Could you check a few things on this model? Use its own coordinates, in mm. Round coordinates to 2 decimals unless told otherwise and drop trailing zeros. Loops run counter-clockwise (first coordinate to the right, second up) from the corner with the lowest first, then second, coordinate; pieces in that order, holes last. Notation, with made-up numbers: (37, 42) - (65, 42) arc R16 cw to (65, 57) - close; hole circle Ø3 at (-23.75, -22). An arc over 180 degrees is marked (long way). Use one line per item in the form item = value.
```python
from build123d import *

# Parameters (mm, degrees)
SKETCH1_R           = 40.64
SKETCH1_R_2         = 27.686
SKETCH1_R_3         = 3.556
SKETCH1_R_4         = 2.794
BOSS_EXTRUDE1_DEPTH = 2.794
SKETCH2_W           = 3.048
SKETCH2_H           = 48.134172809
CUT_EXTRUDE1_DEPTH  = 14.097


with BuildPart() as part:
    # Sketch1 → Boss-Extrude1 (new body)
    with BuildSketch(Plane.XY):
        Circle(SKETCH1_R)
        Circle(SKETCH1_R_2, mode=Mode.SUBTRACT)
        with Locations((0, 34.036)):
            Circle(SKETCH1_R_3, mode=Mode.SUBTRACT)
        with Locations((34.036, 0)):
            Circle(SKETCH1_R_3, mode=Mode.SUBTRACT)
        with Locations((0, -34.036)):
            Circle(SKETCH1_R_3, mode=Mode.SUBTRACT)
        with Locations((-34.036, 0)):
            Circle(SKETCH1_R_3, mode=Mode.SUBTRACT)
        with Locations((24.067086404, 24.067086404)):
            Circle(SKETCH1_R_4, mode=Mode.SUBTRACT)
        with Locations((24.067086404, -24.067086404)):
            Circle(SKETCH1_R_4, mode=Mode.SUBTRACT)
        with Locations((-24.067086404, -24.067086404)):
            Circle(SKETCH1_R_4, mode=Mode.SUBTRACT)
        with Locations((-24.067086404, 24.067086404)):
            Circle(SKETCH1_R_4, mode=Mode.SUBTRACT)
    extrude(amount=BOSS_EXTRUDE1_DEPTH)

    # Sketch2 → Cut-Extrude1 (cut)
    with BuildSketch(Plane.XY.offset(2.794)):
        with Locations((-24.067086404, 24.067086405)):
            Rectangle(SKETCH2_W, SKETCH2_H)
    extrude(amount=-CUT_EXTRUDE1_DEPTH, mode=Mode.SUBTRACT)


solid = part.part
```
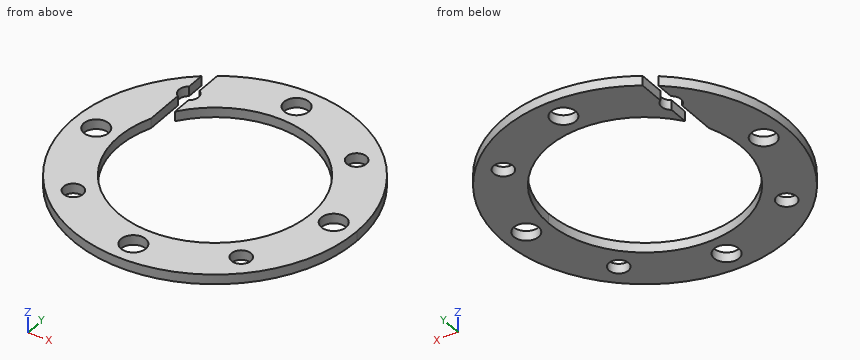
1. If we section it at C-C, the plane y = -12: Write out the boundary of the cut face in (x, z).
Solution:
outline = (-38.83, 0) - (-24.95, 0) - (-24.95, 2.79) - (-38.83, 2.79) - close; (24.95, 0) - (38.83, 0) - (38.83, 2.79) - (24.95, 2.79) - close
2. If we section it at A-A, the plane x = 0: Write out the boundary of the cut face in (y, z), plus the area to 3 significant figures.
Solution:
outline = (-40.64, 0) - (-37.59, 0) - (-37.59, 2.79) - (-40.64, 2.79) - close; (-30.48, 0) - (-27.69, 0) - (-27.69, 2.79) - (-30.48, 2.79) - close; (27.69, 0) - (30.48, 0) - (30.48, 2.79) - (27.69, 2.79) - close; (37.59, 0) - (40.64, 0) - (40.64, 2.79) - (37.59, 2.79) - close
area = 32.6 mm^2
3. Please list where these lines run through material, in increasing order: line 1 along Y through (x, z) = (0, 1.1); line 2 along X through (y, z) = (-2, 1.3); line 3 along X through (y, z) = (7, 1.65).
Solution:
line_1 = -40.64 to -37.59, -30.48 to -27.69, 27.69 to 30.48, 37.59 to 40.64
line_2 = -40.59 to -36.98, -31.1 to -27.61, 27.61 to 31.1, 36.98 to 40.59
line_3 = -40.03 to -26.79, 26.79 to 40.03
4. For P1, Ø1.5, axis at y = 18.5, z = 1.5, coming from the +X side; P2, Ø0.8, axis at y = 19, z = 1.5, coming from the -X side, each with a flat end and sliding along its axis, tell me the tip position at first contact or that it passes through.
Solution:
P1 = 36.56
P2 = -36.13
5. If we section it at B-B, the plane x = 18.5: Write out the boundary of the cut face in (y, z), plus the area to 3 significant figures.
Solution:
outline = (-36.19, 0) - (-20.6, 0) - (-20.6, 2.79) - (-36.19, 2.79) - close; (20.6, 0) - (36.19, 0) - (36.19, 2.79) - (20.6, 2.79) - close
area = 87.1 mm^2
6. If we section it at D-D, the plane z = 1.9: Write out the boundary of the cut face in (x, y), plus the area to 3 significant figures.
Solution:
outline = (-25.59, 10.56) - (-25.59, 21.73) arc R2.79 cw to (-25.59, 26.41) - (-25.59, 31.57) arc R40.64 ccw (long way) to (-22.54, 33.81) - (-22.54, 26.41) arc R2.79 cw to (-22.54, 21.73) - (-22.54, 16.07) arc R27.69 cw (long way) to start; hole circle Ø7.11 at (-34.04, 0); hole circle Ø5.59 at (-24.07, -24.07); hole circle Ø7.11 at (0, -34.04); hole circle Ø7.11 at (0, 34.04); hole circle Ø5.59 at (24.07, -24.07); hole circle Ø5.59 at (24.07, 24.07); hole circle Ø7.11 at (34.04, 0)
area = 2,480 mm^2
